```python
from build123d import *

# Parameters (mm, degrees)
SKETCH1_W                          = 75
SKETCH1_H                          = 50.00000000000001
BE_MAIN_UPRIGHT_BODY_DEPTH         = 221
SKETCH19_R                         = 62.5
BOSS_EXTRUDE1_DEPTH                = 50
SKETCH4_R                          = 35
CE_THROUGH_HOLE_DEPTH              = 236.04733565816056
SKETCH2_R                          = 50
CE_INNER_BEARING_DEPTH             = 16
SKETCH3_R                          = 55
CE_OUTER_BEARING_DEPTH             = 13
BE_CALIPER_MOUNT_V2_DEPTH          = 10
BE_TIE_ROD_MOUNT_V2_DEPTH          = 60.00000000000001
BE_TIE_ROD_MOUNT_V2_DEPTH_BACK     = 9.999999999999996
SKETCH32_R                         = 1.7000000000000146
BE_TEMP_SENSOR_MOUNT_V3_DEPTH      = 10
CE_CALIPER_HOLES_REACH             = 255.863
SKETCH26_R                         = 4.199999999999994
SKETCH26_R_2                       = 4.1999999999999975
CE_CALIPER_HOLES_DIRECTION_2_REACH = 255.863
SKETCH12_R                         = 4.0000000000000036
SKETCH12_R_2                       = 4
CE_TOP_CLEVIS_HOLES_DEPTH          = 252.68750278067682
CE_TOP_CLEVIS_SPACE_DEPTH          = 35
CE_BOTTOM_CLEVIS_SPACE_DEPTH       = 252.68750278067682
SKETCH15_W                         = 25.000000000000004
SKETCH15_H                         = 5
CE_EXPAND_BOTTOM_CLEVIS_DEPTH      = 252.68750278067682
CE_WIDEN_BOTTOM_CLEVIS_DEPTH       = 249.87031277664735
CE_WIDEN_BOTTOM_CLEVIS_DEPTH_BACK  = 249.87031277664735
SKETCH16_W                         = 10.00755403153164
SKETCH16_H                         = 17
CHAMFER1_SIZE                      = 20
CHAMFER2_SIZE                      = 30
CUT_EXTRUDE1_REACH                 = 180.963
SKETCH28_R                         = 4.000000000000007
CUT_EXTRUDE2_REACH                 = 262.905
FILLET2_R                          = 15
FILLET3_R                          = 5


with BuildPart() as part:
    # Sketch1 → BE - main upright body (new body)
    with BuildSketch(Plane(origin=(0, 0, 0), x_dir=(1, 0, 0), z_dir=(0, 1, 0))):
        Rectangle(SKETCH1_W, SKETCH1_H)
    extrude(amount=BE_MAIN_UPRIGHT_BODY_DEPTH)

    # Sketch19 → Boss-Extrude1 (add)
    with BuildSketch(Plane.XY.offset(25)):
        with Locations((0, 110.5)):
            Circle(SKETCH19_R)
    extrude(amount=-BOSS_EXTRUDE1_DEPTH)

    # Sketch4 → CE - Through hole (cut, through all)
    with BuildSketch(Plane.XY.offset(25)):
        with Locations((6.57e-15, 110.5)):
            Circle(SKETCH4_R)
    extrude(amount=-CE_THROUGH_HOLE_DEPTH, mode=Mode.SUBTRACT)

    # Sketch2 → CE - Inner bearing (cut)
    with BuildSketch(Plane.XY.offset(25)):
        with Locations((5.2e-15, 110.5)):
            Circle(SKETCH2_R)
    extrude(amount=-CE_INNER_BEARING_DEPTH, mode=Mode.SUBTRACT)

    # Sketch3 → CE - Outer bearing (cut)
    with BuildSketch(Plane(origin=(0, 0, -25), x_dir=(-1, 0, 0), z_dir=(0, 0, -1))):
        with Locations((0, 110.5)):
            Circle(SKETCH3_R)
    extrude(amount=-CE_OUTER_BEARING_DEPTH, mode=Mode.SUBTRACT)

    # Sketch23 → BE - caliper mount v2 (add, symmetric)
    with BuildSketch(Plane.XY):
        with BuildLine():
            Line((35.05710874811726, 146.15107468538196), (62.54897572629606, 174.1087311459216))
            ThreePointArc((62.54897572629606, 174.1087311459216), (76.02582114581824, 157.1746136728197), (85.02821067036592, 137.4934887074417))
            Line((85.02821067036592, 137.4934887074417), (47.65614773889368, 125.62916331753813))
            ThreePointArc((47.65614773889368, 125.62916331753813), (42.610537560783285, 136.65993288946052), (35.05710874811726, 146.15107468538196))
        make_face()
        with BuildLine():
            Line((35.05710874811726, 74.84892531461804), (62.54897572629606, 46.89126885407838))
            ThreePointArc((62.54897572629606, 46.89126885407838), (76.02582114581824, 63.82538632718028), (85.02821067036592, 83.50651129255829))
            Line((85.02821067036592, 83.50651129255829), (47.65614773889368, 95.37083668246188))
            ThreePointArc((47.65614773889368, 95.37083668246188), (42.61053756078329, 84.34006711053948), (35.05710874811726, 74.84892531461804))
        make_face()
    extrude(amount=BE_CALIPER_MOUNT_V2_DEPTH, both=True)

    # Sketch24 → BE - tie rod mount v2 (add, two sides: drawn at the far end of the back side and taken through both)
    with BuildSketch(Plane.XY.offset(-BE_TIE_ROD_MOUNT_V2_DEPTH_BACK)):
        with BuildLine():
            Line((-35.21675994796843, 75.00662288866886), (-81.12210695526274, 28.74070304926003))
            ThreePointArc((-81.12210695526274, 28.74070304926003), (-98.11223118223046, 50.172817344210976), (-109.57006459783258, 75.00662288866886))
            Line((-109.57006459783258, 75.00662288866886), (-47.56659814757113, 95.0916016190039))
            ThreePointArc((-47.56659814757113, 95.0916016190039), (-42.592519144130065, 84.31074050384561), (-35.21675994796843, 75.00662288866886))
        make_face()
    extrude(amount=BE_TIE_ROD_MOUNT_V2_DEPTH + BE_TIE_ROD_MOUNT_V2_DEPTH_BACK)

    # Sketch32 → BE - temp sensor mount v3 (add, symmetric)
    with BuildSketch(Plane.XY):
        with BuildLine():
            Line((-40.308968964609726, 148.60437176531212), (-80.09470245298189, 148.60437176531215))
            ThreePointArc((-80.09470245298189, 148.60437176531215), (-84.35510834631509, 144.34396587197895), (-80.09470245298189, 140.08355997864578))
            Line((-80.09470245298189, 140.08355997864578), (-40.30896896460972, 140.08355997864575))
            Line((-40.30896896460972, 140.08355997864575), (-40.308968964609726, 148.60437176531212))
        make_face()
        with Locations((-76.1523345656343, 144.34396587197895)):
            Circle(SKETCH32_R, mode=Mode.SUBTRACT)
        with Locations((-66.1523345656343, 144.34396587197895)):
            Circle(SKETCH32_R, mode=Mode.SUBTRACT)
    extrude(amount=BE_TEMP_SENSOR_MOUNT_V3_DEPTH, both=True)

    # Sketch26 → CE - caliper holes (cut, up to next)
    with BuildSketch(Plane.XY, mode=Mode.PRIVATE) as ce_caliper_holes_sk1:
        with Locations(Location((68.41158901726085, 68.50000000000001, 0), (0, 0, 180))):
            Circle(SKETCH26_R)
    ce_caliper_holes_tool1 = extrude(ce_caliper_holes_sk1.sketch, amount=-CE_CALIPER_HOLES_REACH, mode=Mode.PRIVATE) & part.part
    # Sketch26 → CE - caliper holes (cut, up to next)
    with BuildSketch(Plane.XY, mode=Mode.PRIVATE) as ce_caliper_holes_sk2:
        with Locations(Location((68.41158901726085, 152.49999999999997, 0), (0, 0, 180))):
            Circle(SKETCH26_R_2)
    ce_caliper_holes_tool2 = extrude(ce_caliper_holes_sk2.sketch, amount=-CE_CALIPER_HOLES_REACH, mode=Mode.PRIVATE) & part.part
    add(ce_caliper_holes_tool1.solids().sort_by_distance((68.411589, 68.5, 0))[0], mode=Mode.SUBTRACT)
    add(ce_caliper_holes_tool2.solids().sort_by_distance((68.411589, 152.5, 0))[0], mode=Mode.SUBTRACT)

    # Sketch26 → CE - caliper holes direction 2 (cut, up to next)
    with BuildSketch(Plane.XY, mode=Mode.PRIVATE) as ce_caliper_holes_direction_2_sk1:
        with Locations(Location((68.41158901726085, 68.50000000000001, 0), (0, 0, 180))):
            Circle(SKETCH26_R)
    ce_caliper_holes_direction_2_tool1 = extrude(ce_caliper_holes_direction_2_sk1.sketch, amount=CE_CALIPER_HOLES_DIRECTION_2_REACH, mode=Mode.PRIVATE) & part.part
    # Sketch26 → CE - caliper holes direction 2 (cut, up to next)
    with BuildSketch(Plane.XY, mode=Mode.PRIVATE) as ce_caliper_holes_direction_2_sk2:
        with Locations(Location((68.41158901726085, 152.49999999999997, 0), (0, 0, 180))):
            Circle(SKETCH26_R_2)
    ce_caliper_holes_direction_2_tool2 = extrude(ce_caliper_holes_direction_2_sk2.sketch, amount=CE_CALIPER_HOLES_DIRECTION_2_REACH, mode=Mode.PRIVATE) & part.part
    add(ce_caliper_holes_direction_2_tool1.solids().sort_by_distance((68.411589, 68.5, 0))[0], mode=Mode.SUBTRACT)
    add(ce_caliper_holes_direction_2_tool2.solids().sort_by_distance((68.411589, 152.5, 0))[0], mode=Mode.SUBTRACT)

    # Sketch12 → CE - top clevis holes (cut, through all)
    with BuildSketch(Plane.XY.offset(25)):
        with Locations((-12.5, 201)):
            Circle(SKETCH12_R)
        with Locations((12.5, 201)):
            Circle(SKETCH12_R_2)
    extrude(amount=-CE_TOP_CLEVIS_HOLES_DEPTH, mode=Mode.SUBTRACT)

    # Sketch13 → CE - top clevis space (cut)
    with BuildSketch(Plane.XY.offset(25)):
        Polygon((-27.499999999999968, 191.00000000000006), (27.500000000000032, 191.00000000000006), (27.500000000000032, 211.00000000000003), (-27.499999999999968, 211.00000000000006), align=None)
    extrude(amount=-CE_TOP_CLEVIS_SPACE_DEPTH, mode=Mode.SUBTRACT)

    # Sketch14 → CE - bottom clevis space (cut, through all)
    with BuildSketch(Plane.XY.offset(25)):
        Polygon((-22.48000000000002, 4.500000000000011), (2.5199999999999796, 4.500000000000011), (2.51999999999998, 16.50000000000001), (-22.48000000000002, 16.50000000000001), align=None)
    extrude(amount=-CE_BOTTOM_CLEVIS_SPACE_DEPTH, mode=Mode.SUBTRACT)

    # Sketch15 → CE - expand bottom clevis (cut, through all)
    with BuildSketch(Plane.XY.offset(25)):
        with Locations((-9.98000000000002, 19.00000000000001)):
            Rectangle(SKETCH15_W, SKETCH15_H)
    extrude(amount=-CE_EXPAND_BOTTOM_CLEVIS_DEPTH, mode=Mode.SUBTRACT)

    # Sketch16 → CE - widen bottom clevis (cut, two sides: drawn at the far end of the back side and taken through both)
    with BuildSketch(Plane(origin=(2.5199999999999796, 4.500000000000011, 25), x_dir=(1, 0, 0), z_dir=(0, 0, 1)).offset(-CE_WIDEN_BOTTOM_CLEVIS_DEPTH_BACK)):
        with Locations((5.00377701576582, 8.5)):
            Rectangle(SKETCH16_W, SKETCH16_H)
    extrude(amount=CE_WIDEN_BOTTOM_CLEVIS_DEPTH + CE_WIDEN_BOTTOM_CLEVIS_DEPTH_BACK, mode=Mode.SUBTRACT)

    # Chamfer1
    chamfer1_edges = [part.edges().sort_by_distance(p)[0] for p in [
        (-42.592519144130065, 84.31074050384561, 60.00000000000001),
    ]]
    chamfer(chamfer1_edges, length=CHAMFER1_SIZE)

    # Chamfer2
    chamfer2_edges = [part.edges().sort_by_distance(p)[0] for p in [
        (-98.11223118223045, 50.17281734421098, -9.999999999999996),
    ]]
    chamfer(chamfer2_edges, length=CHAMFER2_SIZE)

    # Cut-Extrude1: up to this plane
    cut_extrude1_end = Plane(origin=(-35.21675994796843, 75.00662288866886, -9.999999999999996), z_dir=(0.7098675422266223, -0.7043351989593695, 0))
    # Sketch28 → Cut-Extrude1 (cut, up to the surface)
    with BuildSketch(Plane(origin=(-32.39528914978471, 100.00609166249728, 0), x_dir=(0.951331962951422, 0.3081679676199239, 0), z_dir=(-0.3081679676199238, 0.9513319629514219, 0)), mode=Mode.PRIVATE) as cut_extrude1_sk1:
        with Locations(Location((-50.230429584814566, -49.15, 0), (0, 0, 180))):
            Circle(SKETCH28_R)
    cut_extrude1_tool1 = split(extrude(cut_extrude1_sk1.sketch, amount=-CUT_EXTRUDE1_REACH, mode=Mode.PRIVATE), bisect_by=cut_extrude1_end, keep=Keep.BOTH, mode=Mode.PRIVATE)
    add(cut_extrude1_tool1.solids().sort_by_distance((-80.181102, 84.526682, 49.15))[0], mode=Mode.SUBTRACT)

    # Sketch29 → Cut-Extrude2 (cut, up to next)
    with BuildSketch(Plane.XY.offset(60.00000000000001), mode=Mode.PRIVATE) as cut_extrude2_sk1:
        with BuildLine():
            Line((-70.0705275210271, 78.4190759215617), (-93.07971814036846, 70.96563612779761))
            ThreePointArc((-93.07971814036846, 70.96563612779761), (-86.14562004973435, 57.53083914090252), (-77.28611251700346, 45.279936615492176))
            Line((-77.28611251700346, 45.279936615492176), (-60.250857228734134, 62.4489987616883))
            ThreePointArc((-60.250857228734134, 62.4489987616883), (-65.64812771052121, 70.13432343060958), (-70.0705275210271, 78.4190759215617))
        make_face()
    cut_extrude2_tool1 = extrude(cut_extrude2_sk1.sketch, amount=-CUT_EXTRUDE2_REACH, mode=Mode.PRIVATE) & part.part
    add(cut_extrude2_tool1.solids().sort_by_distance((-76.449162, 63.492991, 60))[0], mode=Mode.SUBTRACT)

    # Fillet2
    # the kernel refuses this fillet: 15 mm, written as the material it takes off along each edge
    with BuildSketch(Plane(origin=(-81.12210695526272, 28.740703049260055, -23.23718779420447), x_dir=(0.70433519895937, 0.7098675422266219, 0), z_dir=(0, 0, 1))) as fillet2_piece_1:
        with BuildLine():
            CenterArc((16.129396420502527, 15.000000000000002), FILLET2_R, 171.38829576022673, 98.6117042397733)
            ThreePointArc((1.2985092148828912, 17.246059815362816), (0.3250860863217871, 8.647437558840888), (0, 0))
            Line((0, 0), (16.12939642050253, 3.6e-16))
        make_face()
    extrude(amount=126.47437558840895, mode=Mode.SUBTRACT)
    with BuildSketch(Plane(origin=(-109.57006459783257, 75.00662288866886, 103.23718779420446), x_dir=(0.3787247076655996, -0.9255093709971856, 0), z_dir=(0, 0, -1))) as fillet2_piece_2:
        with BuildLine():
            CenterArc((16.16866645235697, -14.957662051341691), FILLET2_R, 85.69414788011332, 98.61170423977336)
            Line((1.2110044010152803, -16.083870716666514), (0, 0))
            ThreePointArc((0, 0), (8.6474375588409, 0.3250860863217989), (17.29487511768179, -4.5e-16))
        make_face()
    extrude(amount=126.47437558840892, mode=Mode.SUBTRACT)

    # Fillet3
    fillet3_edges = [part.edges().sort_by_distance(p)[0] for p in [
        (-77.28611251700346, 45.279936615492176, 32.976107440368864),
        (-93.07971814036846, 70.96563612779761, 32.976107440368864),
    ]]
    fillet(fillet3_edges, radius=FILLET3_R)


solid = part.part
```
The listing builds one solid part. Answer for the finished solid, in the listing's coordinates (mm). A direction names the side the tool comes from. Coordinates: 2 decimals unless noted, no trailing zeros. Write each loop counter-clockwise with the first axis right and the second up, starting at its lowest first coordinate (ties: lowest second). Pieces come first, ordered by that corner, then holes. Notation, with made-up numbers: M 51.25,58 L 110.25,58 A25 cw 110.25,79 Z; hole C 63,87 d6. An arc over 180 degrees is marked long. Use a Markdown table: item, result. Add a question column.
1. Given P1, Ø2, axis at x = -46.5, z = 8, coming from the +Y side; P2, Ø4.5, axis at x = -74, y = 143, coming from the +Z side; P3, Ø10, axis at x = -0.5, y = 204, coming from the +Z side; P4, Ø6.5, axis at x = 68.41, y = 152.5, coming from the +Z side, each flat-ended and moving along its own axis, determine where each tip first touches the part or whether it passes through.
2. Section B-B (x = 0) is taken. Give the vertices of the cut face in (y, z), plus the area to 3 significant figures.
3. Which of the six approach directions +Z, -Z, +X, -X, +Y, -Y give full straight-line access (tool end or side, diameter ignored) to faces 1 (the flat face through (-27.5, 201, 8)), 2 (the flat face through (72.48, 87.49, 0.14)), 3 (the flat face through (-66.88, 55.77, 25.49)), 4 (the flat face through (65, 147, -10))?
4. Section C-C (z = 33) is taken. Give the vertices of the cut face in (x, y), plus the area to 3 significant figures.
5. Section A-A (y = 19) is taken. Give the vertices of the cut face in (x, z).
6. Section D-D (x = 25) is taken. Give the vertices of the cut face in (y, z).
7. Straight lines are drawn through the part: line 1 along Y through (x, z) = (0, -15.75); line 2 along Y through (x, z) = (0, 1.5); line 3 along X through (y, z) = (14, 8). For each, find the intervals that lie inside material, in ascending order. Write a range as [from, to].
8. For a pull along Y with two mould halves and no side action, classify faces 5 (the flat face through (12.528, 13, 0)), 6 (the flat face through (-37.5, 190, 0)), 7 (the flat face through (53.1, 56.5, 0.1)) as +Y half, -Y half, draft (parallel to the pull), parting line (faces both ways), or undercut.
Data:
| question | item | result |
|---|---|---|
| 1 | P1 | stops at y = 153.35 |
| 1 | P2 | stops at z = 10 |
| 1 | P3 | stops at z = -10 |
| 1 | P4 | passes through |
| 2 | outline | M 0,-25 L 4.5,-25 L 4.5,25 L 0,25 Z; M 21.5,-25 L 55.5,-25 L 55.5,-12 L 75.5,-12 L 75.5,9 L 60.5,9 L 60.5,25 L 21.5,25 Z; M 145.5,-12 L 165.5,-12 L 165.5,-25 L 221,-25 L 221,25 L 211,25 L 211,-10 L 191,-10 L 191,25 L 160.5,25 L 160.5,9 L 145.5,9 Z |
| 2 | area | 5,000 mm2 |
| 3 | face 1 | +Z |
| 3 | face 2 | +Z, -Z, +X |
| 3 | face 3 | +Z, -Z |
| 3 | face 4 | -Z, +X, +Y |
| 4 | outline | M -103.02,59 A115.18 ccw -92.45,41.81 A15 ccw -69.76,40.19 L -35.22,75.01 A50 cw -47.57,95.09 L -94.23,79.98 A15 ccw Z; hole M -90.68,65.73 A101.13 ccw -80.88,49.79 A5 ccw -73.33,49.27 L -60.25,62.45 A77.07 cw -70.07,78.42 L -87.73,72.7 A5 ccw Z |
| 4 | area | 1,870 mm2 |
| 5 | outline | M -37.5,-25 L -22.48,-25 L -22.48,25 L -37.5,25 Z; M 12.53,-25 L 37.5,-25 L 37.5,25 L 12.53,25 Z |
| 6 | outline | M 0,-25 L 61.51,-25 L 61.51,-12 L 86.01,-12 L 86.01,9 L 67.2,9 L 67.2,25 L 0,25 Z; M 134.99,-12 L 159.49,-12 L 159.49,-25 L 221,-25 L 221,25 L 211,25 L 211,-10 L 191,-10 L 191,25 L 153.8,25 L 153.8,9 L 134.99,9 Z |
| 7 | line 1 | y = [0, 4.5], [21.5, 55.5], [165.5, 221] |
| 7 | line 2 | y = [0, 4.5], [21.5, 75.5], [145.5, 191], [211, 221] |
| 7 | line 3 | x = [-37.5, -22.48], [12.53, 37.5] |
| 8 | face 5 | undercut |
| 8 | face 6 | draft |
| 8 | face 7 | -Y half |
